```python
from build123d import *

# Parameters (mm, degrees)
CROQUIS1_R              = 4
SALIENTE_EXTRUIR1_DEPTH = 7.5
CROQUIS2_R              = 3.19
CORTAR_EXTRUIR1_DEPTH   = 155.064651655
REDONDEO1_R             = 12
CHAFL_N1_SIZE           = 1
REDONDEO2_R             = 5
CHAFL_N2_SIZE           = 2
CHAFL_N3_SIZE           = 1


with BuildPart() as part:
    # Croquis1 → Saliente-Extruir1 (new, symmetric)
    with BuildSketch(Plane.XY):
        with BuildLine():
            Line((-15, 0), (-15, 55.980762114))
            Line((-15, 55.980762114), (-26.794919243, 100))
            Line((-26.794919243, 100), (-31.794919243, 100))
            Line((-31.794919243, 100), (-31.794919243, 150))
            Line((-31.794919243, 150), (-16.794919243, 150))
            Line((-16.794919243, 150), (15, 55.980762114))
            Line((15, 55.980762114), (15, 0))
            ThreePointArc((15, 0), (0, -15), (-15, 0))
        make_face()
        Circle(CROQUIS1_R, mode=Mode.SUBTRACT)
        with BuildLine():
            Line((9.744122991, 54.61268154), (-2.226582025, 21.723439813))
            ThreePointArc((-2.226582025, 21.723439813), (-7.353433082, 19.332749903), (-9.744122991, 24.459600959))
            Line((-9.744122991, 24.459600959), (2.226582025, 57.348842687))
            ThreePointArc((2.226582025, 57.348842687), (7.353433082, 59.739532597), (9.744122991, 54.61268154))
        make_face(mode=Mode.SUBTRACT)
    extrude(amount=SALIENTE_EXTRUIR1_DEPTH, both=True)

    # Croquis2 → Cortar-Extruir1 (cut, through all)
    with BuildSketch(Plane.XY.offset(7.5)):
        with Locations((-24.794919243, 125)):
            Circle(CROQUIS2_R)
    extrude(amount=-CORTAR_EXTRUIR1_DEPTH, mode=Mode.SUBTRACT)

    # Redondeo1
    redondeo1_edges = [part.edges().sort_by_distance(p)[0] for p in [
        (-15, 55.980762114, 0),
        (15, 55.980762114, 0),
    ]]
    fillet(redondeo1_edges, radius=REDONDEO1_R)

    # Chaflán1
    chafl_n1_edges = [part.edges().sort_by_distance(p)[0] for p in [
        (-4, 0, -7.5),
        (-4, 0, 7.5),
    ]]
    chamfer(chafl_n1_edges, length=CHAFL_N1_SIZE)

    # Redondeo2
    redondeo2_edges = [part.edges().sort_by_distance(p)[0] for p in [
        (-16.794919243, 150, 0),
    ]]
    fillet(redondeo2_edges, radius=REDONDEO2_R)

    # Chaflán2
    chafl_n2_edges = [part.edges().sort_by_distance(p)[0] for p in [
        (15, 27.00331421, -7.5),
        (0, -15, -7.5),
        (-21.101904664, 78.753380342, 7.5),
        (0, -15, 7.5),
        (-15, 27.200466071, -7.5),
        (-15, 27.200466071, 7.5),
        (-0.639069755, 102.226308716, -7.5),
        (-0.639069755, 102.226308716, 7.5),
        (14.840839938, 55.95457851, -7.5),
        (14.840839938, 55.95457851, 7.5),
        (-15.102661664, 55.967246449, -7.5),
        (-15.102661664, 55.967246449, 7.5),
        (-26.088566443, 150, -7.5),
        (-26.088566443, 150, 7.5),
        (-17.467493018, 149.062561222, -7.5),
        (-17.467493018, 149.062561222, 7.5),
        (15, 27.00331421, 7.5),
        (-21.101904664, 78.753380342, -7.5),
    ]]
    chamfer(chafl_n2_edges, length=CHAFL_N2_SIZE)

    # Chaflán3
    chafl_n3_edges = [part.edges().sort_by_distance(p)[0] for p in [
        (7.353433082, 59.739532597, -7.5),
        (-3.758770483, 40.904221823, -7.5),
        (-7.353433082, 19.332749903, -7.5),
        (3.758770483, 38.168060676, -7.5),
        (7.353433082, 59.739532597, 7.5),
        (-3.758770483, 40.904221823, 7.5),
        (-7.353433082, 19.332749903, 7.5),
        (3.758770483, 38.168060676, 7.5),
    ]]
    chamfer(chafl_n3_edges, length=CHAFL_N3_SIZE)


solid = part.part
```
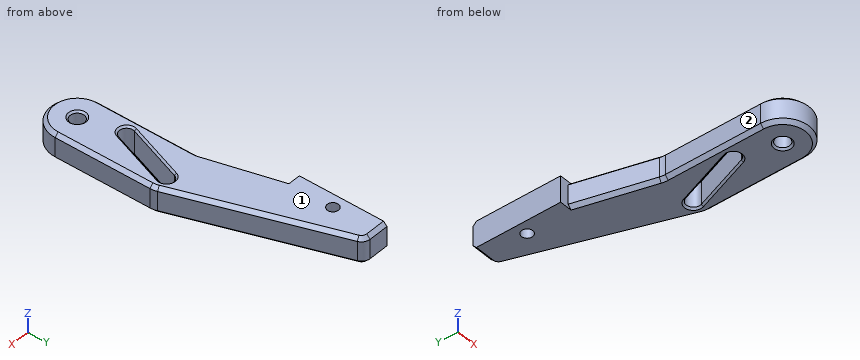
Here's how the part is built. I have some questions about the finished solid (model axes, mm). Face numbers are marked on the shaded views. A direction names the side the tool comes from. Round coordinates to 2 decimals unless told otherwise and drop trailing zeros. Order: outer loops, then holes, each group sorted by start corner. A loop starts at its lowest first (then second) coordinate and runs counter-clockwise, first axis right, second up. Notation, with made-up numbers: M 24,-26 L 79,-26 A24 cw 79,9 Z; hole C -36.5,-21 d8. An arc over 180 degrees is marked long. Answer in a Markdown table with one row per item.
Item 1: Imagine slicing it at C-C, the plane y = 125. Write out the boundary of the cut face in (x, z), and give its area (3 significant figures).
A:
| item | result |
|---|---|
| outline | M -31.79,-7.5 L -27.98,-7.5 L -27.98,7.5 L -31.79,7.5 Z; M -21.6,-7.5 L -10.45,-7.5 L -8.34,-5.5 L -8.34,5.5 L -10.45,7.5 L -21.6,7.5 Z |
| area | 252 mm2 |
Item 2: For the marked faces 1 and 2, which set-ups out of +Z, -Z, +X, -X, +Y, -Y let a thin tool reach every point of the face, with its end or its side?
A:
| item | result |
|---|---|
| face 1 | +Z, +X, -X, +Y, -Y |
| face 2 | +Z, -Z, -X, -Y |
Item 3: I'm going to push flat-ended pins straight in: pin 1 (9 mm diameter, centred on y = 18, z = 0, fed in from -X); pin 2 (5 mm diameter, centred on x = -16, z = 5, fed in from -Y); pin 3 (10 mm diameter, centred on x = -24.79, y = 125, fed in from +Z); pin 4 (7 mm diameter, centred on x = 0, y = 0, fed in from -Z). Where does each tip first touch, or does it pass through?
A:
| item | result |
|---|---|
| pin 1 | stops at x = -15 |
| pin 2 | stops at y = -6.54 |
| pin 3 | stops at z = 7.5 |
| pin 4 | passes through |
Item 4: Imagine slicing it at B-B, the plane y = 13.5. Write out the boundary of the cut face in (x, z).
A:
| item | result |
|---|---|
| outline | M -15,-5.5 L -13,-7.5 L 13,-7.5 L 15,-5.5 L 15,5.5 L 13,7.5 L -13,7.5 L -15,5.5 Z |
Item 5: If I drill on L1, parallel to X at y = 6.5, z = -1; L2, parallel to X at y = 32.5, z = -4.25; L3, parallel to X at y = 58, z = 2, over which ranges is the centre line in solid material (lowest first)? Write a range as from..to.
A:
| item | result |
|---|---|
| L1 | x = -15..15 |
| L2 | x = -15..-6.82, 1.7..15 |
| L3 | x = -15.54..2.53, 9.44..14.32 |
Item 6: Imagine slicing it at A-A, the plane z = -1.5. Write out the boundary of the cut face in (x, y), and give its area (3 significant figures).
A:
| item | result |
|---|---|
| outline | M -31.79,100 L -26.79,100 L -15.41,57.51 A12 cw -15,54.4 L -15,0 A15 ccw 15,0 L 15,54.01 A12 ccw 14.37,57.85 L -15.65,146.6 A5 ccw -20.38,150 L -31.79,150 Z; hole C -24.79,125 d6.38; hole M -9.74,24.46 A4 ccw -2.23,21.72 L 9.74,54.61 A4 ccw 2.23,57.35 Z; hole C 0,0 d8 |
| area | 4,040 mm2 |
